from build123d import *

# Parameters (mm, degrees)
SKETCH1_W           = 16
SKETCH1_H           = 4
SKETCH1_W_2         = 76
SKETCH1_H_2         = 16
SKETCH1_R           = 4.125
BOSS_EXTRUDE1_DEPTH = 10
SKETCH2_W           = 6
SKETCH2_H           = 2.8
CUT_EXTRUDE1_DEPTH  = 10
SKETCH3_R           = 1.55
CUT_EXTRUDE2_DEPTH  = 10
FILLET1_R           = 8
FILLET2_R           = 2
SKETCH4_W           = 38
SKETCH4_H           = 32.700002283
SKETCH4_R           = 1.55
SKETCH4_R_2         = 12.5
BOSS_EXTRUDE2_DEPTH = 10
CUT_EXTRUDE3_DEPTH  = 10
FILLET4_R           = 2


with BuildPart() as part:
    # Sketch1 → Boss-Extrude1 (new body)
    # profile 1 of 3: a face of its own
    with BuildSketch(Plane(origin=(0, 0, 0), x_dir=(1, 0, 0), z_dir=(0, 1, 0))):
        with Locations((-30, -10)):
            Rectangle(SKETCH1_W, SKETCH1_H)
    # profile 2 of 3: a face of its own
    with BuildSketch(Plane(origin=(0, 0, 0), x_dir=(1, 0, 0), z_dir=(0, 1, 0))):
        Rectangle(SKETCH1_W_2, SKETCH1_H_2)
        with Locations(Location((30, 0, 0), (0, 0, 270))):
            Circle(SKETCH1_R, mode=Mode.SUBTRACT)
        with Locations(Location((-30, 2.283e-06, 0), (0, 0, 270))):
            Circle(SKETCH1_R, mode=Mode.SUBTRACT)
    # profile 3 of 3: a face of its own
    with BuildSketch(Plane(origin=(0, 0, 0), x_dir=(1, 0, 0), z_dir=(0, 1, 0))):
        with Locations((30, -10)):
            Rectangle(SKETCH1_W, SKETCH1_H)
    extrude(amount=BOSS_EXTRUDE1_DEPTH)

    # Sketch2 → Cut-Extrude1 (cut)
    with BuildSketch(Plane(origin=(0, 10, 0), x_dir=(1, 0, 0), z_dir=(0, 1, 0))):
        with Locations((-30, -7.999997717)):
            Rectangle(SKETCH2_W, SKETCH2_H)
    cut_extrude1 = extrude(amount=-CUT_EXTRUDE1_DEPTH, mode=Mode.SUBTRACT)

    # Sketch3 → Cut-Extrude2 (cut)
    with BuildSketch(Plane.XY.offset(12)):
        with Locations((-30, 5.258558289)):
            Circle(SKETCH3_R)
    cut_extrude2 = extrude(amount=-CUT_EXTRUDE2_DEPTH, mode=Mode.SUBTRACT)

    # Mirror1: Cut-Extrude1, Cut-Extrude2 across plane
    add(cut_extrude1.mirror(Plane(origin=(0, 0, 0), x_dir=(0, 0, 1), z_dir=(1, 0, 0))), mode=Mode.SUBTRACT)
    add(cut_extrude2.mirror(Plane(origin=(0, 0, 0), x_dir=(0, 0, 1), z_dir=(1, 0, 0))), mode=Mode.SUBTRACT)

    # Fillet1
    fillet1_edges = [part.edges().sort_by_distance(p)[0] for p in [
        (-38, 5, -8),
        (38, 5, -8),
    ]]
    fillet(fillet1_edges, radius=FILLET1_R)

    # Fillet2
    fillet2_edges = [part.edges().sort_by_distance(p)[0] for p in [
        (38, 5, 12),
        (22, 5, 12),
        (22, 5, 8),
        (-22, 5, 8),
        (-22, 5, 12),
        (-38, 5, 12),
    ]]
    fillet(fillet2_edges, radius=FILLET2_R - 0.0001)  # a hair under: the kernel refuses the full size

    # Sketch4 → Boss-Extrude2 (add)
    with BuildSketch(Plane.XZ):
        with Locations((0, -24.350001142)):
            Rectangle(SKETCH4_W, SKETCH4_H)
        with Locations(Location((15.5, -37.200002283, 0), (0, 0, 270))):
            Circle(SKETCH4_R, mode=Mode.SUBTRACT)
        with Locations(Location((-15.5, -37.200002283, 0), (0, 0, 270))):
            Circle(SKETCH4_R, mode=Mode.SUBTRACT)
        with Locations(Location((0, -21.700002283, 0), (0, 0, 270))):
            Circle(SKETCH4_R_2, mode=Mode.SUBTRACT)
    extrude(amount=-BOSS_EXTRUDE2_DEPTH)

    # Sketch4<3> → Cut-Extrude3 (cut)
    with BuildSketch(Plane.XZ):
        with BuildLine():
            ThreePointArc((17.05, -6.200002283), (15.5, -4.650002283), (13.95, -6.200002283))
            Line((13.95, -6.200002283), (15.5, -6.200002283))
            Line((15.5, -6.200002283), (15.5, -7.750002283))
            ThreePointArc((15.5, -7.750002283), (16.596015511, -7.296017794), (17.05, -6.200002283))
        make_face()
        with BuildLine():
            Line((15.5, -6.200002283), (13.95, -6.200002283))
            ThreePointArc((13.95, -6.200002283), (14.403984489, -7.296017794), (15.5, -7.750002283))
            Line((15.5, -7.750002283), (15.5, -6.200002283))
        make_face()
        with BuildLine():
            Line((-15.5, -7.750002283), (-15.5, -6.200002283))
            Line((-15.5, -6.200002283), (-13.95, -6.200002283))
            ThreePointArc((-13.95, -6.200002283), (-16.596015511, -5.103986772), (-15.5, -7.750002283))
        make_face()
        with BuildLine():
            Line((-13.95, -6.200002283), (-15.5, -6.200002283))
            Line((-15.5, -6.200002283), (-15.5, -7.750002283))
            ThreePointArc((-15.5, -7.750002283), (-14.403984489, -7.296017794), (-13.95, -6.200002283))
        make_face()
    extrude(amount=-CUT_EXTRUDE3_DEPTH, mode=Mode.SUBTRACT)

    # Fillet4
    fillet4_edges = [part.edges().sort_by_distance(p)[0] for p in [
        (19, 5, -8),
        (-19, 5, -8),
        (19, 5, -40.700002283),
        (-19, 5, -40.700002283),
    ]]
    fillet(fillet4_edges, radius=FILLET4_R)


solid = part.part
Check sheet for the modelled part. Datum: model origin and axes. Units: mm. A direction names the side the tool comes from. Round coordinates to 2 decimals unless told otherwise and drop trailing zeros. Loops run counter-clockwise (first coordinate to the right, second up) from the corner with the lowest first, then second, coordinate; pieces in that order, holes last.
1. Set-up check for faces 5 (the flat face through (33, 5, 8)), 6 (the cylindrical face through (28.57, 4.66, 10.72)), 7 (the flat face through (0, 5, 8)), 8 (the flat face through (19, 5, -25)), 9 (the flat face through (-26, 5, -8)): record each of +Z, -Z, +X, -X, +Y, -Y from which the full face is reachable in a straight line by a thin tool's end or side.
2. Sectioned sample at D-D on y = 8. Give the number of separate pieces and of enclosed holes in the cut face, and give its area (3 significant figures).
3. Mould release check, pull along Z, two halves, no side actions. Record for faces 1 (the cylindrical face through (-28.57, 4.66, 10.72)), 2 (the cylindrical face through (-22.57, 5.07, 11.4)), 3 (the cylindrical face through (-19.57, 5.07, -8.6)), 4 (the flat face through (28.7, 4, 6.6)): released by +Z, released by -Z, zero draft, split by the parting line, or undercut.
4. Sectioned sample at B-B on z = 2. Record the boundary of the cut face in (x, y), and give its area (3 significant figures).
5. Sectioned sample at A-A on x = 0. Record the boundary of the cut face in (y, z).
6. Gauge pin test, flat ends, axial feed: pin 1 Ø4 at (x, y) = (-30, 5.26) entering from -Z; pin 2 Ø3 at (y, z) = (3.5, -13.5) entering from -X; pin 3 Ø5 at (y, z) = (7, -24) entering from +X. Record the tip position at first contact, or that the pin passes through.
7. Scan lines: probe 1 along X at (y, z) = (2.75, 0) (3 decimals); probe 2 along X at (y, z) = (5, 7); probe 3 along Z at (x, y) = (-31, 7.5). Record each from-to range of solid material in increasing order.
8. Sectioned sample at C-C on z = -25.5. Record the boundary of the cut face in (x, y).
Recorded:
1. face 5: +Y, -Y
1. face 6: +Z
1. face 7: +Z, +Y, -Y
1. face 8: -Z, +X, +Y, -Y
1. face 9: -Z, -X, +Y, -Y
2. separate pieces: 1
2. enclosed holes: 9
2. area: 1,900 mm2
3. face 1: zero draft
3. face 2: released by +Z
3. face 3: released by -Z
3. face 4: undercut
4. outline: (-38, 0) - (-33.61, 0) - (-33.61, 10) - (-38, 10) - close; (-26.39, 0) - (26.39, 0) - (26.39, 10) - (-26.39, 10) - close; (33.61, 0) - (38, 0) - (38, 10) - (33.61, 10) - close
4. area: 616 mm2
5. outline: (0, -40.7) - (10, -40.7) - (10, -34.2) - (0, -34.2) - close; (0, -9.2) - (10, -9.2) - (10, 8) - (0, 8) - close
6. pin 1: stops at z = -8
6. pin 2: stops at x = -19
6. pin 3: stops at x = 19
7. probe 1: x = -38 to -34.125, -25.875 to 25.875, 34.125 to 38
7. probe 2: x = -38 to -33, -27 to 27, 33 to 38
7. probe 3: z = -7.94 to -4, 4 to 6.6, 9.4 to 12
8. outline: (-19, 0) - (-11.91, 0) - (-11.91, 10) - (-19, 10) - close; (11.91, 0) - (19, 0) - (19, 10) - (11.91, 10) - close
